Here's the drawing with two shaded views (mm, measured from the low corner). I have some questions. A direction names the side the tool comes from. Round coordinates to 2 decimals unless told otherwise and drop trailing zeros. Order: outer loops, then holes, each group sorted by start corner. A loop starts at its lowest first (then second) coordinate and runs counter-clockwise, first axis right, second up. Notation, with made-up numbers: (-17.5, -34.5) -> (41.5, -34.5) arc R18 cw to (41.5, -9.5) -> close; hole circle Ø4 at (-3, 38.5). An arc over 180 degrees is marked (long way). One line per question, with ' | ' between items.
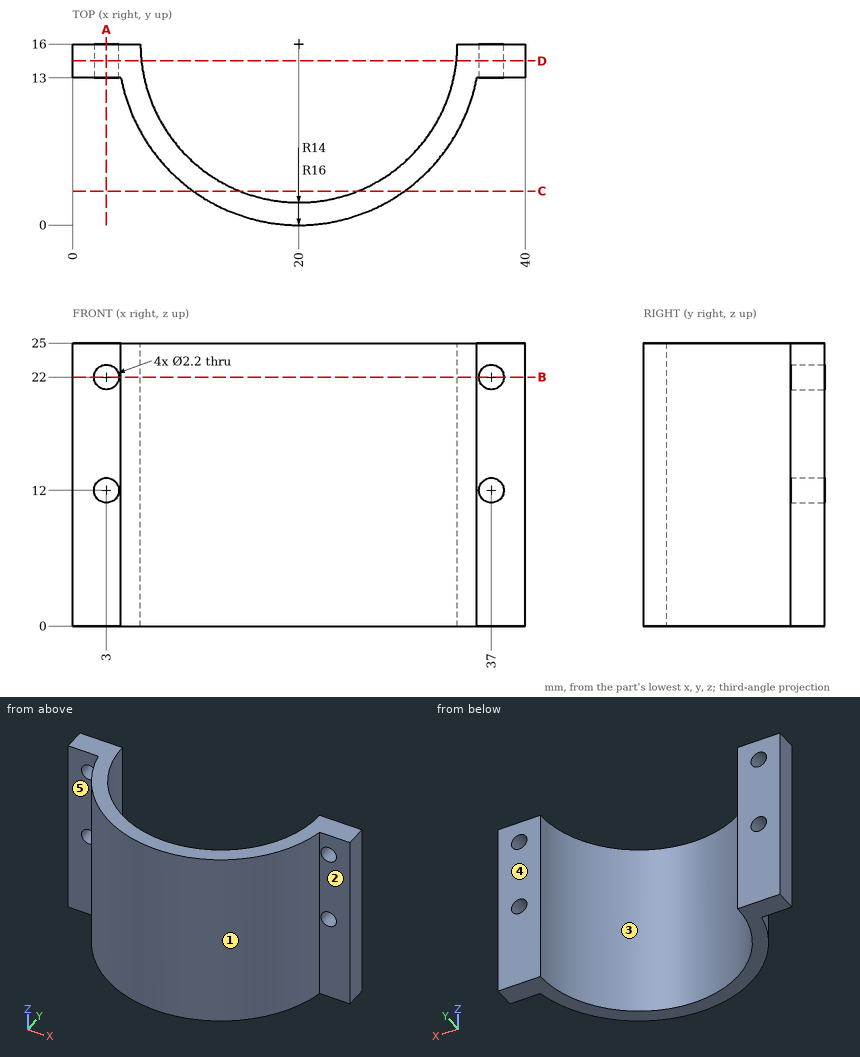
1. If we mould it in two halves opening along X, with no side actions, what happens to the marked faces 1, 2 and 3? For each: pulls with the +X half, pulls with the -X half, needs draft (parallel to the pull), parting line crosses it, or undercut.
From the geometry:
face 1: parting line crosses it | face 2: needs draft | face 3: undercut
2. On a 3-axis mill with a long thin cutter (end or side, diameter ignored), from which of +Z, -Z, +X, -X, +Y, -Y can I reach the whole of each face in a straight line? I mean the marked faces 4 and 5. Say none if no direction works.
From the geometry:
face 4: +Z, -Z, +X, -X, +Y | face 5: +Z, -Z, -X, -Y
3. I'm going to push flat-ended pins straight in: pin 1 (4.5 mm diameter, centred on x = 1.5, z = 16, fed in from -Y); pin 2 (2.5 mm diameter, centred on x = 37, z = 12, fed in from +Y); pin 3 (2 mm diameter, centred on y = 5, z = 10.5, fed in from -X); pin 4 (4 mm diameter, centred on y = 6.5, z = 8, fed in from +X). Where does each tip first touch, or does it pass through?
From the geometry:
pin 1: stops at y = 13 | pin 2: stops at y = 16 | pin 3: stops at x = 7.51 | pin 4: stops at x = 34.13
4. I need wall thicknesses on probe 1 along Z at (x, y) = (37, 13.9); probe 2 along X at (y, z) = (15.5, 14); probe 3 along X at (y, z) = (12.5, 19.75). Which ranges of each line are inside material? Lowest first, please.
From the geometry:
probe 1: z = 0 to 10.9, 13.1 to 20.9, 23.1 to 25 | probe 2: x = 0 to 6.01, 33.99 to 40 | probe 3: x = 4.39 to 6.44, 33.56 to 35.61
5. I want a section at B-B on z = 22. List the corners of the cut face in (x, y) for me.
From the geometry:
outline: (0, 13) -> (1.9, 13) -> (1.9, 16) -> (0, 16) -> close; (4.1, 13) -> (4.28, 13) arc R16 ccw to (35.72, 13) -> (35.9, 13) -> (35.9, 16) -> (34, 16) arc R14 cw to (6, 16) -> (4.1, 16) -> close; (38.1, 13) -> (40, 13) -> (40, 16) -> (38.1, 16) -> close
6. I want a section at C-C on y = 3. List the corners of the cut face in (x, z) for me.
From the geometry:
outline: (10.67, 0) -> (14.8, 0) -> (14.8, 25) -> (10.67, 25) -> close; (25.2, 0) -> (29.33, 0) -> (29.33, 25) -> (25.2, 25) -> close
7. I want a section at D-D on y = 14.5. List the corners of the cut face in (x, z) for me.
From the geometry:
outline: (0, 0) -> (6.08, 0) -> (6.08, 25) -> (0, 25) -> close; (33.92, 0) -> (40, 0) -> (40, 25) -> (33.92, 25) -> close; hole circle Ø2.2 at (3, 12); hole circle Ø2.2 at (3, 22); hole circle Ø2.2 at (37, 12); hole circle Ø2.2 at (37, 22)
8. I want a section at A-A on x = 3. List the corners of the cut face in (y, z) for me, and give its area (3 significant figures).
From the geometry:
outline: (13, 0) -> (16, 0) -> (16, 10.9) -> (13, 10.9) -> close; (13, 13.1) -> (16, 13.1) -> (16, 20.9) -> (13, 20.9) -> close; (13, 23.1) -> (16, 23.1) -> (16, 25) -> (13, 25) -> close | area: 61.8 mm²
